from build123d import *

# Parameters (mm, degrees)
F0_R     = 7
F1_DEPTH = 1
F2_W     = 9.4
F2_H     = 9.4
F3_DEPTH = 0.9
F4_SIZE2 = 0.5
F4_SIZE  = 0.5
F5_R     = 1.5


with BuildPart() as f1:
    # F0 (on Top) → F1 (new body)
    with BuildSketch(Plane.XY):
        Circle(F0_R)
        with BuildLine():
            ThreePointArc((2.03101, 3.475), (0, -4.025), (-2.03101, 3.475))
            Line((-2.03101, 3.475), (2.03101, 3.475))
        make_face(mode=Mode.SUBTRACT)
    extrude(amount=-F1_DEPTH)

    # F2 (on face) → F3 (join)
    with BuildSketch(Plane.XY):
        Rectangle(F2_W, F2_H)
        with BuildLine():
            Line((-2.03101, 3.475), (2.03101, 3.475))
            ThreePointArc((2.03101, 3.475), (0, -4.025), (-2.03101, 3.475))
        make_face(mode=Mode.SUBTRACT)
    extrude(amount=F3_DEPTH)

    # F4
    f4_edges = [f1.edges().sort_by_distance(p)[0] for p in [
        (0, -4.025, -1),
        (-7, 0, -1),
        (0, 3.475, -1),
        (0, -4.025, 0.9),
        (0, 3.475, 0.9),
    ]]
    chamfer(f4_edges, length=F4_SIZE, length2=F4_SIZE2)

    # F5
    f5_edges = [f1.edges().sort_by_distance(p)[0] for p in [
        (-4.7, 4.7, 0.45),
        (4.7, 4.7, 0.45),
        (4.7, -4.7, 0.45),
        (-4.7, -4.7, 0.45),
    ]]
    fillet(f5_edges, radius=F5_R)


solid = f1.part
Read the model definition and answer for the solid it produces. Units are mm, in the model's axes. A direction names the side the tool comes from. Round coordinates to 2 decimals unless told otherwise and drop trailing zeros. Order: outer loops, then holes, each group sorted by start corner. A loop starts at its lowest first (then second) coordinate and runs counter-clockwise, first axis right, second up. Notation, with made-up numbers: (-29.75, 87.25) - (8.25, 87.25) arc R25 cw to (8.25, 126.25) - close; hole circle Ø3 at (52, 14.5). An arc over 180 degrees is marked (long way). Use one line per item in the form item = value. Start each with the question number.
(1) Determine the mould class of faces 1 (the face through (6.466, -2.681, -0.246)), 2 (the face through (4.7, 0, 0.4)), 3 (the face through (0, -4.7, 0.4)), 4 (the face through (0.147, -4.022, -0.056)) for opening direction Y: +Y half, -Y half, draft (parallel to the pull), parting line (faces both ways), or undercut.
(2) Find the intervals of material crossed by line 1 along Y through (x, z) = (0, 0.15) (3 decimals); line 2 along Y through (x, z) = (0, -0.2) (3 decimals); line 3 along X through (y, z) = (0, 0.2) (3 decimals), in increasing order. Write a range as from..to.
(3) Flat-ended cylindrical pins translate along their axes: pin 1 Ø0.7 at (x, z) = (-1, 0.5) entering from -Y; pin 2 Ø3 at (x, y) = (5.5, -5.5) entering from +Z. Find the tip coordinate at first contact, or state that the pin passes through.
(4) The part is cut by section A-A (x = 0). Give the vertices of the cut face in (y, z) (3 decimals), then the cut area to 3 significant figures.
(5) The part is cut by section D-D (z = -0.25). Give the vertices of the cut face in (x, y) (3 decimals), then the cut area to 3 significant figures.
(6) The part is cut by section C-C (z = 0.6). Give the vertices of the cut face in (x, y) (3 decimals), then the cut area to 3 significant figures.
(7) For faces 5 (the face through (0, 5, 0)), 6 (the face through (-4.27, 4.25, 0.46)), 7 (the face through (0, 4.7, 0.4)), determine the directions among +Z, -Z, +X, -X, +Y, -Y from which every point of the face is accessible in a straight line to the end or side of a thin tool.
(8) The part is cut by section B-B (y = 0). Give the vertices of the cut face in (x, z) (3 decimals).
Checked values:
q1.face_1 = parting line
q1.face_2 = draft
q1.face_3 = -Y half
q1.face_4 = undercut
q2.line_1 = -4.7..-4.025, 3.475..4.7
q2.line_2 = -7..-4.025, 3.475..7
q2.line_3 = -4.7..-4.025, 4.025..4.7
q3.pin_1 = -4.7
q3.pin_2 = 0
q4.outline = (-7, -0.5) - (-6.5, -1) - (-4.525, -1) - (-4.025, -0.5) - (-4.025, 0.4) - (-4.525, 0.9) - (-4.7, 0.9) - (-4.7, 0) - (-7, 0) - close; (3.475, -0.5) - (3.975, -1) - (6.5, -1) - (7, -0.5) - (7, 0) - (4.7, 0) - (4.7, 0.9) - (3.975, 0.9) - (3.475, 0.4) - close
q4.area = 7.46 mm^2
q5.outline = circle Ø14 at (0, 0); hole (-2.031, 3.475) arc R4.025 ccw (long way) to (2.031, 3.475) - close
q5.area = 105 mm^2
q6.outline = (-4.7, -3.2) arc R1.5 ccw to (-3.2, -4.7) - (3.2, -4.7) arc R1.5 ccw to (4.7, -3.2) - (4.7, 3.2) arc R1.5 ccw to (3.2, 4.7) - (-3.2, 4.7) arc R1.5 ccw to (-4.7, 3.2) - close; hole (-2.084, 3.675) arc R4.225 ccw (long way) to (2.084, 3.675) - close
q6.area = 31.9 mm^2
q7.face_5 = +Z
q7.face_6 = +Z, -X, +Y
q7.face_7 = +Z, +X, -X, +Y
q8.outline = (-7, -0.5) - (-6.5, -1) - (-4.525, -1) - (-4.025, -0.5) - (-4.025, 0.4) - (-4.525, 0.9) - (-4.7, 0.9) - (-4.7, 0) - (-7, 0) - close; (4.025, -0.5) - (4.525, -1) - (6.5, -1) - (7, -0.5) - (7, 0) - (4.7, 0) - (4.7, 0.9) - (4.525, 0.9) - (4.025, 0.4) - close
